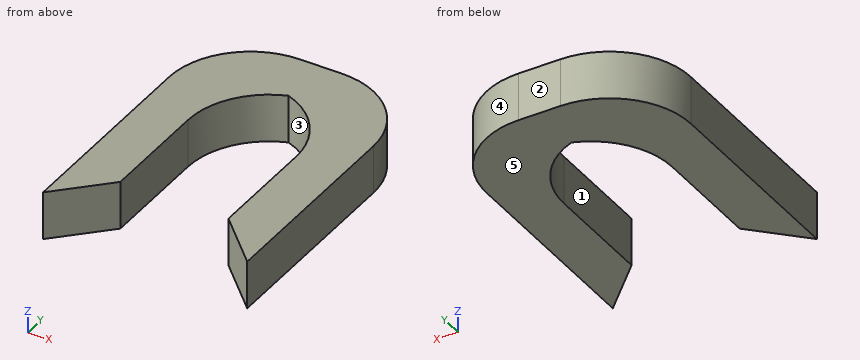
from build123d import *

# Parameters (mm, degrees)
F0_W        = 4.5
F0_H        = 2
F1_DEPTH    = 2
F2_T1_DEPTH = 2
F2_T3_DEPTH = 18.8994949366
F3_SIZE     = 1.99999


# Not quite as in the source:
# - a fillet or chamfer that OpenCascade refuses, or shapes differently, is made with other operations: its cross-section is extruded or revolved along the edge and cut away or added
# - a fillet or chamfer is up to 0.001 mm smaller than in the source, because OpenCascade refuses the exact size


with BuildPart() as f1:
    # F0 (on Top) → F1 (new body)
    with BuildSketch(Plane.XY):
        Polygon((0, 12), (0, 0), (2, 0), (2, 10), (2, 12), align=None)
        Polygon((6.5, 12), (6.5, 10), (6.5, 0), (8.5, 0), (8.5, 12), align=None)
        with Locations((4.25, 11)):
            Rectangle(F0_W, F0_H)
    extrude(amount=F1_DEPTH)

    # F2: fillet of radius 3.3798989873 on 4 edges, made by hand

    # F2_s2 → F2_t1 (join)
    with BuildSketch(Plane.XY):
        with BuildLine():
            ThreePointArc((3.1201010127, 10), (5.5100505063, 9.0100505063), (6.5, 6.6201010127))
            Line((6.5, 6.6201010127), (6.5, 10))
            Line((6.5, 10), (3.1201010127, 10))
        make_face()
        with BuildLine():
            ThreePointArc((2, 6.6201010127), (2.9899494937, 9.0100505063), (5.3798989873, 10))
            Line((5.3798989873, 10), (2, 10))
            Line((2, 10), (2, 6.6201010127))
        make_face()
    extrude(amount=F2_T1_DEPTH)

    # F2_s4 → F2_t3 (cut)
    with BuildSketch(Plane.XY.offset(-8.4497474683)):
        with BuildLine():
            ThreePointArc((0, 8.6201010127), (0.9899494937, 11.0100505063), (3.3798989873, 12))
            Line((3.3798989873, 12), (0, 12))
            Line((0, 12), (0, 8.6201010127))
        make_face()
        with BuildLine():
            ThreePointArc((5.1201010127, 12), (7.5100505063, 11.0100505063), (8.5, 8.6201010127))
            Line((8.5, 8.6201010127), (8.5, 12))
            Line((8.5, 12), (5.1201010127, 12))
        make_face()
    extrude(amount=F2_T3_DEPTH, mode=Mode.SUBTRACT)

    # F3 (size 2 in the source; OpenCascade refuses exactly that, so slightly less here)
    f3_edges = [f1.edges().sort_by_distance(p)[0] for p in [
        (2, 0, 1),
        (6.5, 0, 1),
    ]]
    chamfer(f3_edges, length=F3_SIZE)


solid = f1.part
Design review of the part built by this model. Coordinates are the model's own, in mm. Face numbers are marked on the shaded views. A direction names the side the tool comes from. Give positions to 0.01 mm unless a question says otherwise; leave off trailing zeros. Order: outer loops, then holes, each group sorted by start corner. A loop starts at its lowest first (then second) coordinate and runs counter-clockwise, first axis right, second up. Notation, with made-up numbers: (-19, 86) - (31, 86) arc R16 ccw to (31, 106) - close; hole circle Ø11 at (35.5, 47.5). An arc over 180 degrees is marked (long way). Write item = value, one per line. Start each with the question number.
Q1. To check wall thickness, follow L1, parallel to X at y = 5.25, z = 1; L2, parallel to X at y = 1, z = 0.35; L3, parallel to Y at x = 1.5, z = 1.45. State the ranges of each line that lie inside material, in increasing order. Write a range as from..to.
Q2. Clearance check with a flat-ended pin moving along its axis: pin 1 Ø2 at (x, y) = (1, 6.5) entering from -Z. State where the tip first meets the part, or that it passes through.
Q3. Tool access review of the marked faces 1 and 2: name each direction out of +Z, -Z, +X, -X, +Y, -Y from which nothing blocks a thin tool from reaching the whole face with its end or side.
Q4. We need section A-A on y = 3.25. State the section outline as (x, z) points.
Q5. We need section D-D on x = 0.5. State the section outline as (y, z) points, plus the area to 3 significant figures.
Q6. We need section C-C on y = 7.75. State the section outline as (x, z) points, plus the area to 3 significant figures.
Q7. Mouldability with a two-part tool opening along X and no side actions: class the marked faces 3, 4 and 5 as released by +X, released by -X, zero draft, split by the parting line, or undercut.
Working result:
q1.L1 = 0..2, 6.5..8.5
q1.L2 = 0..1, 7.5..8.5
q1.L3 = 1.5..11.43
q2.pin_1 = 0
q3.face_1 = +Z, -Z, -Y
q3.face_2 = +Z, -Z, +X, -X, +Y
q4.outline = (0, 0) - (2, 0) - (2, 2) - (0, 2) - close; (6.5, 0) - (8.5, 0) - (8.5, 2) - (6.5, 2) - close
q5.outline = (0.5, 0) - (10.39, 0) - (10.39, 2) - (0.5, 2) - close
q5.area = 19.8 mm²
q6.outline = (0, 0) - (2.19, 0) - (2.19, 2) - (0, 2) - close; (6.31, 0) - (8.5, 0) - (8.5, 2) - (6.31, 2) - close
q6.area = 8.78 mm²
q7.face_3 = undercut
q7.face_4 = released by +X
q7.face_5 = zero draft
